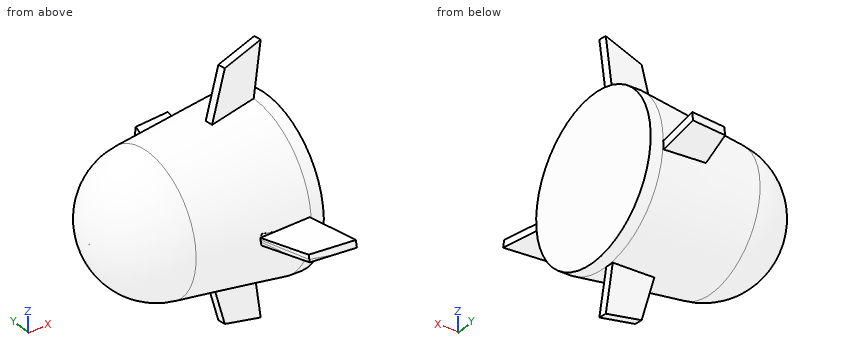
from build123d import *

# Parameters (mm, degrees)
BOSS_EXTRUDE1_DEPTH  = 4
BOSS_EXTRUDE5_DEPTH  = 0.5
CIRPATTERN27_COUNT   = 2
CIRPATTERN28_COUNT   = 2
CIRPATTERN28_ANGLE   = 270
MIRROR5_COPY_1_DEPTH = 4
MIRROR5_COPY_2_DEPTH = 0.5
CUT_EXTRUDE1_DEPTH   = 7.5
CUT_EXTRUDE5_DEPTH   = 7.5
CUT_EXTRUDE8_DEPTH   = 7.5
CUT_EXTRUDE9_DEPTH   = 7.5
SCALE1_SCALE         = 0.78
SKETCH35_R           = 32.4987
BOSS_EXTRUDE6_DEPTH  = 5


with BuildPart() as part:
    # Sketch1 → Revolve1 (revolve)
    with BuildSketch(Plane.XY, mode=Mode.PRIVATE) as revolve1_sk:
        with BuildLine():
            Line((68.355271076, -5.571052632), (68.355271076, 36.093947368))
            Line((68.355271076, 36.093947368), (13.656115926, 29.428947368))
            ThreePointArc((13.656115926, 29.428947368), (-8.192658078, 17.861941693), (-16.644728924, -5.370084567))
            Line((-16.644728924, -5.370084567), (-16.644728924, -5.571052632))
            Line((-16.644728924, -5.571052632), (68.355271076, -5.571052632))
        make_face()
    revolve(revolve1_sk.sketch.rotate(Axis((-16.644728924, -5.571052632, 0), (1, 0, 0)), 90), axis=Axis((-16.644728924, -5.571052632, 0), (1, 0, 0)))



with BuildPart() as body_2:
    # Sketch3 → Boss-Extrude1 (new body)
    with BuildSketch(Plane(origin=(0.689359663, -0.083997315, -5.279598975), x_dir=(0.984180627017453, -0.11992075309071235, 0.13041283058690828), z_dir=(0.12945535873547723, -0.01577391759705046, -0.9914597791228399))):
        Polygon((48.907006258, 38.621427836), (59.41626027, 62.048150042), (80.536298945, 65.037658628), (72.938516553, 38.621427836), align=None)
    boss_extrude1 = extrude(amount=BOSS_EXTRUDE1_DEPTH)


with BuildPart() as part_1:
    add(part.part)

    add(body_2.part)  # Boss-Extrude5 merges body 2
    # Sketch12 → Boss-Extrude5 (add)
    with BuildSketch(Plane(origin=(-4.671405547, -38.337874984, 0), x_dir=(0.9926581468470392, -0.12095372461483828, 0), z_dir=(0.12095372461483828, 0.9926581468470392, 0))):
        Polygon((49.183787896, -1.098502146), (73.010063784, -4.232519427), (73.531715107, -0.266680311), (49.705439218, 2.86733697), align=None)
    boss_extrude5 = extrude(amount=BOSS_EXTRUDE5_DEPTH)

    # CirPattern27: Boss-Extrude1, Boss-Extrude5 ×2 about axis
    cirpattern27_axis = Axis((0, -5.571052632, 0), (1, 0, 0))
    add([boss_extrude1.rotate(cirpattern27_axis, i * 360 / CIRPATTERN27_COUNT) for i in range(1, CIRPATTERN27_COUNT)])
    add([boss_extrude5.rotate(cirpattern27_axis, i * 360 / CIRPATTERN27_COUNT) for i in range(1, CIRPATTERN27_COUNT)])

    # CirPattern28: Boss-Extrude1, Boss-Extrude5 ×2 about axis
    cirpattern28_axis = Axis((0, -5.571052632, 0), (1, 0, 0))
    add([boss_extrude1.rotate(cirpattern28_axis, i * CIRPATTERN28_ANGLE / (CIRPATTERN28_COUNT - 1)) for i in range(1, CIRPATTERN28_COUNT)])
    add([boss_extrude5.rotate(cirpattern28_axis, i * CIRPATTERN28_ANGLE / (CIRPATTERN28_COUNT - 1)) for i in range(1, CIRPATTERN28_COUNT)])

    # Mirror5: Boss-Extrude1, Boss-Extrude5 across plane
    add(boss_extrude1.mirror(Plane.XY))
    add(boss_extrude5.mirror(Plane.XY))

    # Mirror5 copy 1 sketch → Mirror5 copy 1 (add)
    with BuildSketch(Plane(origin=(0.689359663, -10.850651607, 5.487055317), x_dir=(0.984180627017453, 0.13041283058690448, -0.1199207530907165), z_dir=(0.12945535873547723, -0.9914597791228404, -0.01577391759701894))):
        Polygon((48.907006258, -38.621427836), (59.41626027, -62.048150042), (80.536298945, -65.037658628), (72.938516553, -38.621427836), align=None)
    extrude(amount=MIRROR5_COPY_1_DEPTH)

    # Mirror5 copy 2 sketch → Mirror5 copy 2 (add)
    with BuildSketch(Plane(origin=(-4.671405547, -5.571052632, -32.766822353), x_dir=(0.9926581468470392, -3.849360784322416e-15, -0.12095372461483828), z_dir=(0.12095372461483828, 3.155393511496951e-14, 0.9926581468470392))):
        Polygon((49.183787896, 1.098502146), (73.010063784, 4.232519427), (73.531715107, 0.266680311), (49.705439218, -2.86733697), align=None)
    extrude(amount=MIRROR5_COPY_2_DEPTH)

    # Sketch19 → Cut-Extrude1 (cut)
    with BuildSketch(Plane(origin=(1.207181098, -0.147092985, -9.245438092), x_dir=(-0.9915852481222116, -0.002136148499024363, -0.1294377556047779), z_dir=(0.12945535873547703, -0.01577391759705043, -0.99145977912284))):
        Polygon((-67.679175208, -47.235274194), (-71.995880368, -74.381353157), (-48.207029253, -72.13480707), (-43.827344507, -44.302074699), align=None)
    extrude(amount=CUT_EXTRUDE1_DEPTH, mode=Mode.SUBTRACT)

    # Sketch25 → Cut-Extrude5 (cut)
    with BuildSketch(Plane(origin=(0.689359663, -0.083997315, -5.279598975), x_dir=(0.9915852481222117, 0.0021361484990243696, 0.12943775560477816), z_dir=(-0.12945535873547726, 0.015773917597050467, 0.9914597791228399))):
        Polygon((50.891173425, -68.699745189), (71.995880368, -74.381353157), (67.745856954, -47.027055514), (43.827344507, -44.302074699), align=None)
    extrude(amount=CUT_EXTRUDE5_DEPTH, mode=Mode.SUBTRACT)

    # Sketch27 → Cut-Extrude8 (cut)
    with BuildSketch(Plane(origin=(27.301219353, 8.554612251, 3.42863066), x_dir=(-0.1138420069613441, -0.034629872676622354, 0.9928951452038701), z_dir=(-0.9474716659737562, -0.29688244383743123, -0.11898847304688671))):
        Polygon((-1.047061464, -81.100132743), (-2.40192559, -55.459928446), (-6.401425806, -55.574995755), (-5.041488706, -81.311203845), (-3.533903508, -81.231540942), align=None)
    extrude(amount=CUT_EXTRUDE8_DEPTH, mode=Mode.SUBTRACT)

    # Sketch28 → Cut-Extrude9 (cut)
    with BuildSketch(Plane(origin=(-13.685744002, -51.305630722, -0.970692032), x_dir=(-0.9662265281220836, 0.25764897067882825, 0.00482744873453606), z_dir=(-0.25769418750233414, -0.9660536410379842, -0.018277537163565623))):
        Polygon((-89.283438439, -2.656910088), (-88.769166907, -6.623772053), (-66.015638627, -3.548604791), (-66.551372854, 0.415356464), align=None)
    extrude(amount=CUT_EXTRUDE9_DEPTH, mode=Mode.SUBTRACT)


with BuildPart() as part_2:
    # Scale1: scaled about (34.142034643, -5.554496793, -1.7178e-05)
    add(part_1.part.scale(SCALE1_SCALE).moved(Location((7.511247621, -1.221989294, -3.779e-06))))

    # Sketch35 → Boss-Extrude6 (add)
    with BuildSketch(Plane(origin=(60.828359062, 0, 0), x_dir=(0, 0, -1), z_dir=(1, 0, 0))):
        with Locations((3.778e-06, -5.567410349)):
            Circle(SKETCH35_R)
    extrude(amount=BOSS_EXTRUDE6_DEPTH)


solid = part_2.part
Model file for the job. Use its own axes, mm. Give positions to 0.01 mm unless a question says otherwise; leave off trailing zeros. Order: outer loops, then holes, each group sorted by start corner. A loop starts at its lowest first (then second) coordinate and runs counter-clockwise, first axis right, second up. Notation, with made-up numbers: (0, 40) - (55, 40) arc R29 cw to (55, 70) - close; hole circle Ø1 at (-23, -8.75). An arc over 180 degrees is marked (long way). One line per item, written item: value.
Item 1: Slice it at A-A (z = 47). List the corners of the cut face in (x, y).
Response values:
outline: (47.1, -3.77) - (47.48, -6.87) - (63.09, -4.83) - (62.69, -1.73) - close
Item 2: Slice it at C-C (x = 21). List the corners of the cut face in (y, z), then the cut area to 3 significant figures.
Response values:
outline: circle Ø55.29 at (-5.57, 0)
area: 2,400 mm2
Item 3: Wall check: line 1 (Y direction, x = 5, z = -14); line 2 (Z direction, x = 28.5, y = 14); line 3 (Z direction, x = 36.5, y = -22.5). Give the ranges that are in metal, low to high.
Response values:
line 1: -22.44 to 11.31
line 2: -20.8 to 20.8
line 3: -24.2 to 24.2
Item 4: Pin check, flat tips, straight feed: pin 1 Ø10 at (x, z) = (29, 0) entering from -Y; pin 2 Ø10 at (x, y) = (48, 13) entering from +Z. Stop position of each tip, or through.
Response values:
pin 1: y = -34.8
pin 2: z = 27.89
Item 5: Slice it at B-B (y = 32). List the corners of the cut face in (x, z), then the cut area to 3 significant figures.
Response values:
outline: (44.21, -1.27) - (61.21, -3.49) - (61.6, -0.39) - (44.6, 1.83) - close
area: 53.5 mm2
Item 6: Slice it at D-D (x = 32). List the corners of the cut face in (y, z), then the cut area to 3 significant figures.
Response values:
outline: circle Ø57.97 at (-5.57, 0)
area: 2,640 mm2
